Verification items for this drawing (mm, ordinates from the low corner). Coordinates: 2 decimals unless noted, no trailing zeros. Order: outer loops, then holes, each group sorted by start corner. A loop starts at its lowest first (then second) coordinate and runs counter-clockwise, first axis right, second up. Notation, with made-up numbers: (26, 15) -> (35, 15) arc R28 ccw to (35, 49) -> close; hole circle Ø8 at (32, 60). An arc over 180 degrees is marked (long way). Write item = value, one per line. Start each with the question number.
1. Cross-section at A-A on y = 80. Record the cut outline in (x, z).
2. Go/stop test with a flat-tipped pin: P1, Ø1, axis at x = 107.5, z = 1, coming from the -Y side. Record where the tip stops, or that it passes through.
3. Cross-section at B-B on x = 80. Record the cut outline in (y, z).
4. Thickness scan on line 1 along X through (y, z) = (139.5, 1.05) (1 decimal); line 2 along Y through (x, z) = (80, 1); line 3 along Y through (x, z) = (63, 1.65) (1 decimal). Record the ranges inside material, lowest first. Write a range as from..to.
5. Cross-section at C-C on z = 0.6. Record the cut outline in (x, y) (1 decimal).
6. Cross-section at D-D on x = 127. Record the cut outline in (y, z) (1 decimal).
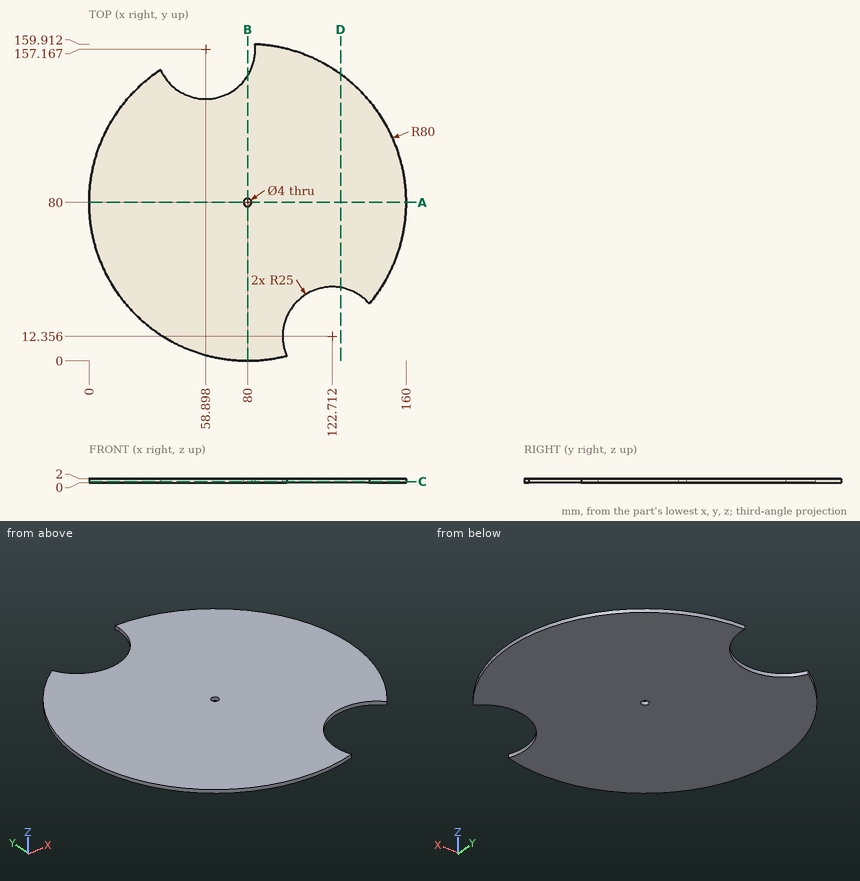
Worked out:
q1.outline = (0, 0) -> (78, 0) -> (78, 2) -> (0, 2) -> close; (82, 0) -> (160, 0) -> (160, 2) -> (82, 2) -> close
q2.P1 = 31.8
q3.outline = (0, 0) -> (78, 0) -> (78, 2) -> (0, 2) -> close; (82, 0) -> (143.76, 0) -> (143.76, 2) -> (82, 2) -> close
q4.line_1 = 26.5..41.2, 76.6..133.5
q4.line_2 = 0..78, 82..143.76
q4.line_3 = 1.8..132.5
q5.outline = (36.1, 146.9) arc R80 ccw to (99.7, 2.5) arc R25 cw to (141.5, 28.8) arc R80 ccw to (83.7, 159.9) arc R25 cw to start; hole circle Ø4 at (80, 80)
q6.outline = (37, 0) -> (144.7, 0) -> (144.7, 2) -> (37, 2) -> close
